Autodesk Inventor part; units mm, degrees
ref_plane "YZ Plane" through (0, 0, 0) normal (1, 0, 0) x (0, 1, 0)
ref_plane "XZ Plane" through (0, 0, 0) normal (0, 1, 0) x (-1, 0, 0)
ref_plane "XY Plane" through (0, 0, 0) normal (0, 0, 1) x (1, 0, 0)
sketch "Skizze1" plane through (0, 0, 0) normal (0, 0, 1) x (1, 0, 0)
  line L0 (-16, 20) -> (16, 20)
  line L1 (16, 20) -> (16, -20)
  line L2 (16, -20) -> (-16, -20)
  line L3 (-16, -20) -> (-16, 20)
  line L4 (-16, 20) -> (16, -20) construction
  line L5 (16, 20) -> (-16, -20) construction
  point P0 (0, 0)
  dimension "d0" = 32
  dimension "d1" = 40
extrude "Extrusion1" add sketch "Skizze1" along normal blind 15
sketch "Skizze2" plane through (-16, -20, 0) normal (0, -1, 0) x (1, 0, 0)
  line L0 (0, 15) -> (32, 15)
  line L1 (0, 0) -> (0, 15)
  line L2 (32, 0) -> (0, 0)
  line L3 (32, 0) -> (32, 15)
  line L4 (32, 15) -> (0, 15)
  circle A0 centre (16, 15) radius 10
  point P0 (16, 0)
  dimension "d4" = 20
extrude "Extrusion2" cut sketch "Skizze2" against normal blind 15 contours A0 L0 | L0 A0
sketch "Skizze3" plane through (-16, -5, 0) normal (0, -1, 0) x (1, 0, 0)
  line L0 (0, 0) -> (0, 15)
  line L1 (32, 0) -> (0, 0)
  line L2 (32, 0) -> (32, 15)
  line L3 (26, 15) -> (32, 15)
  line L4 (0, 15) -> (6, 15)
  line L5 (6, 15) -> (26, 15)
  circle A0 centre (16, 15) radius 10.5
  point P0 (16, 0)
  dimension "d7" = 21
extrude "Extrusion3" cut sketch "Skizze3" against normal blind 5 contours A0 L3 L5 L4 | L4 L5 L3 A0
sketch "Skizze4" plane through (-16, 0, 0) normal (0, -1, 0) x (1, 0, 0)
  line L0 (5.5, 15) -> (26.5, 15)
  circle A0 centre (16, 15) radius 12.5
  point P0 (16, 0)
  dimension "d10" = 25
extrude "Extrusion4" cut sketch "Skizze4" against normal through all
sketch "Skizze5" plane through (0, 0, 15) normal (0, 0, 1) x (1, 0, 0)
  line L0 (-16, 20) -> (-16, -20)
  line L1 (-16, -20) -> (-10, -20)
  line L2 (-10, -20) -> (-10, -5)
  line L3 (10, -5) -> (10, -20)
  line L4 (10, -20) -> (16, -20)
  line L5 (16, -20) -> (16, 20)
  circle A0 centre (-13, -13) radius 1.8
  circle A1 centre (13, -13) radius 1.8
  point P0 (0, 0)
  dimension "d13" = 3.6
  dimension "d14" = 3.6
  dimension "d15" = 7
  dimension "d16" = 7
  dimension "d17" = 3
  dimension "d18" = 3
extrude "Extrusion5" cut sketch "Skizze5" against normal through all
Input: part model. Units: mm. Frame: model coordinates. A direction names the side the tool comes from. Round coordinates to 2 decimals unless told otherwise and drop trailing zeros. Write each loop counter-clockwise with the first axis right and the second up, starting at its lowest first coordinate (ties: lowest second). Pieces come first, ordered by that corner, then holes. Notation, with made-up numbers: M 53,55.5 L 62,55.5 A17 cw 62,87.5 Z; hole C 17,75.5 d9. An arc over 180 degrees is marked long. Write each question's results on one line, items separated by ' | '.
Q1. Access query for faces 1 (the face through (-2, -5, 5)), 2 (the face through (-11.283, -12.459, 7.605)). Directions: +Z, -Z, +X, -X, +Y, -Y. A direction counts if a zero-diameter tool reaches every point of the face in a straight line with its end or side. Return the directions, or none.
Results:
face 1: +Z, +Y | face 2: +Z, -Z
Q2. Section query A-A (z = 7.25). Return loops of the section in (x, y), and give its area (3 significant figures).
Results:
outline: M -16,-20 L -6.32,-20 L -6.32,-5 L -7.08,-5 L -7.08,0 L -9.81,0 L -9.81,20 L -16,20 Z; M 6.32,-20 L 16,-20 L 16,20 L 9.81,20 L 9.81,0 L 7.08,0 L 7.08,-5 L 6.32,-5 Z; hole C -13,-13 d3.6; hole C 13,-13 d3.6 | area: 607 mm^2
Q3. Section query D-D (z = 1). Return loops of the section in (x, y).
Results:
outline: M -16,-20 L 16,-20 L 16,20 L -16,20 Z; hole C -13,-13 d3.6; hole C 13,-13 d3.6
Q4. Pin query (flat end, axial travel): P1, Ø6, axis at x = 13, y = -13, coming from the +Z side; P2, Ø3, axis at x = -8, y = 4, coming from the +Z side. Return the tip coordinate at first contact, or that it passes through.
Results:
P1: stops at z = 15 | P2: stops at z = 6.88
Q5. Draft query along Y for faces 3 (the face through (11.2, -12.92, 7.6)), 4 (the face through (14, 0, 15)), 5 (the face through (0, 20, 2)). Return one class per face: released by +Y, released by -Y, zero draft, split by the parting line, or undercut.
Results:
face 3: undercut | face 4: zero draft | face 5: released by +Y
Q6. Line query: line 1 along Y through (x, z) = (-13, 10.5); line 2 along X through (y, z) = (12.5, 4.25); line 3 along X through (y, z) = (16, 8). Output: solid intervals per line, ascending.
Results:
line 1: y = -20 to -14.8, -11.2 to 20 | line 2: x = -16 to -6.38, 6.38 to 16 | line 3: x = -16 to -10.36, 10.36 to 16
Q7. Section query B-B (x = 13). Return loops of the section in (y, z), and give its area (3 significant figures).
Results:
outline: M -20,0 L -14.8,0 L -14.8,15 L -20,15 Z; M -11.2,0 L 20,0 L 20,15 L -11.2,15 Z | area: 546 mm^2
Q8. Section query C-C (y = -13). Return loops of the section in (x, z).
Results:
outline: M -16,0 L -14.8,0 L -14.8,15 L -16,15 Z; M -11.2,0 L 11.2,0 L 11.2,15 L 10,15 A10 cw -10,15 L -11.2,15 Z; M 14.8,0 L 16,0 L 16,15 L 14.8,15 Z
